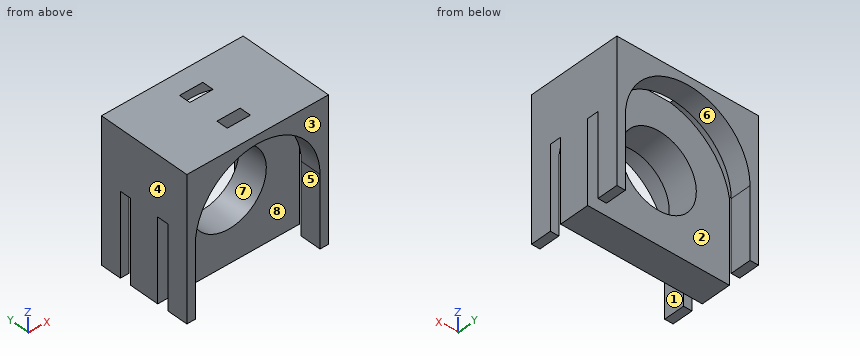
from build123d import *

# Parameters (mm, degrees)
SKETCH1_W           = 15
SKETCH1_H           = 15
BOSS_EXTRUDE1_DEPTH = 5
SKETCH2_W           = 15
SKETCH2_H           = 2.5
BOSS_EXTRUDE2_DEPTH = 15
CUT_EXTRUDE1_START  = -7.5
CUT_EXTRUDE1_DEPTH  = 31
SKETCH4_R           = 7.6
CUT_EXTRUDE2_DEPTH  = 1.2
SKETCH5_R           = 6.6
CUT_EXTRUDE3_DEPTH  = 23.2125
CUT_EXTRUDE4_START  = 1.2
SKETCH6_R           = 7.6
CUT_EXTRUDE4_DEPTH  = 1.2
SKETCH7_R           = 6.6
CUT_EXTRUDE5_DEPTH  = 23.2125
SKETCH8_R           = 4
CUT_EXTRUDE6_DEPTH  = 23.2125


with BuildPart() as part:
    # Sketch1 → Boss-Extrude1 (new body)
    with BuildSketch(Plane(origin=(0, 0, 0), x_dir=(1, 0, 0), z_dir=(0, 1, 0))):
        with Locations((7.5, -7.5)):
            Rectangle(SKETCH1_W, SKETCH1_H)
    extrude(amount=BOSS_EXTRUDE1_DEPTH)

    # Sketch2 → Boss-Extrude2 (add)
    with BuildSketch(Plane.XY.offset(15)):
        with Locations((7.5, 6.25)):
            Rectangle(SKETCH2_W, SKETCH2_H)
        with Locations((7.5, -1.25)):
            Rectangle(SKETCH2_W, SKETCH2_H)
    extrude(amount=-BOSS_EXTRUDE2_DEPTH)

    # Sketch3 → Cut-Extrude1 (cut)
    with BuildSketch(Plane(origin=(0, 0, 0), x_dir=(-1, 0, 0), z_dir=(0, 0, -1)).offset(CUT_EXTRUDE1_START)):
        Polygon((-14.1, 7.5), (-14.1, 5.2875), (-15.1, 5.2875), (-15.1, 4.0875), (-7.5, 4.0875), (0.1, 4.0875), (0.1, 5.2875), (-0.9, 5.2875), (-0.9, 7.5), align=None)
    cut_extrude1 = extrude(amount=CUT_EXTRUDE1_DEPTH, mode=Mode.SUBTRACT)

    # Sketch4 → Cut-Extrude2 (cut)
    with BuildSketch(Plane(origin=(0, 4.0875, 0), x_dir=(1, 0, 0), z_dir=(0, 1, 0))):
        with Locations((7.5, -7.5)):
            Circle(SKETCH4_R)
    extrude(amount=CUT_EXTRUDE2_DEPTH, mode=Mode.SUBTRACT)

    # Sketch5 → Cut-Extrude3 (cut, through all)
    with BuildSketch(Plane(origin=(0, 4.0875, 0), x_dir=(1, 0, 0), z_dir=(0, 1, 0))):
        with Locations((7.5, -7.5)):
            Circle(SKETCH5_R)
    extrude(amount=CUT_EXTRUDE3_DEPTH, mode=Mode.SUBTRACT)

    # Mirror1: Cut-Extrude1 across plane
    add(cut_extrude1.mirror(Plane(origin=(0, 2.5, 0), x_dir=(0, 0, 1), z_dir=(0, -1, 0))), mode=Mode.SUBTRACT)

    # Sketch6 → Cut-Extrude4 (cut)
    with BuildSketch(Plane.XZ.offset(-0.9125).offset(CUT_EXTRUDE4_START)):
        with Locations((7.5, 7.5)):
            Circle(SKETCH6_R)
    extrude(amount=-CUT_EXTRUDE4_DEPTH, mode=Mode.SUBTRACT)

    # Sketch7 → Cut-Extrude5 (cut, through all)
    with BuildSketch(Plane.XZ.offset(-0.9125)):
        with Locations((7.5, 7.5)):
            Circle(SKETCH7_R)
    extrude(amount=CUT_EXTRUDE5_DEPTH, mode=Mode.SUBTRACT)

    # Sketch8 → Cut-Extrude6 (cut, through all)
    with BuildSketch(Plane(origin=(0, 4.0875, 0), x_dir=(1, 0, 0), z_dir=(0, 1, 0))):
        with Locations(Location((7.5, -7.5, 0), (0, 0, 270))):
            Circle(SKETCH8_R)
    extrude(amount=-CUT_EXTRUDE6_DEPTH, mode=Mode.SUBTRACT)


solid = part.part
For this review, take the finished solid that the model builds, in its own axes (mm). Face numbers are marked on the shaded views. A direction names the side the tool comes from. Round coordinates to 2 decimals unless told otherwise and drop trailing zeros. Write each loop counter-clockwise with the first axis right and the second up, starting at its lowest first coordinate (ties: lowest second). Pieces come first, ordered by that corner, then holes. Notation, with made-up numbers: (52, -12.75) - (87, -12.75) arc R5 ccw to (87, -4.75) - close; hole circle Ø2 at (45.5, 31.25). An arc over 180 degrees is marked (long way). Write item = value, one per line. Start each with the question number.
1. Wall thickness on L1, parallel to X at y = 5.5, z = 4.75; L2, parallel to X at y = 2.5, z = 7.5; L3, parallel to Y at x = 13.5, z = 4.5: over which ranges is each line inside the solid? List them lowest first.
2. Consider section D-D on y = 0.25. State the section outline as (x, z) points.
3. Consider section A-A on x = 7.5. State the section outline as (y, z) points.
4. Draft analysis for pull direction Y (two halves, no side actions). For the marked faces 1, 2 and 3, state which applies: released by +Y, released by -Y, zero draft, split by the parting line, or undercut.
5. Consider section C-C on x = 5.5. State the section outline as (y, z) points, plus the area to 3 significant figures.
6. Consider section B-B on z = 10.25. State the section outline as (x, y) points.
7. For pin 1 Ø9 at (x, z) = (7.5, 7.5) entering from +Y; pin 2 Ø4.5 at (x, z) = (6, 9) entering from -Y, all flat-tipped, find the tip position at first contact; note any pin that passes through.
8. For the marked faces 4, 5, 6, 7 and 8, list the 3-axis set-ups (+Z, -Z, +X, -X, +Y, -Y) from which the entire face can be reached by the end or side of a thin tool; tool diameter is ignored.
Evaluation:
q1.L1 = 0 to 0.9, 14.1 to 15
q1.L2 = 0 to 3.5, 11.5 to 15
q1.L3 = 0.91 to 4.09
q2.outline = (0, 8.73) arc R7.6 cw to (6.27, 15) - (0, 15) - close; (8.73, 15) arc R7.6 cw to (15, 8.73) - (15, 15) - close
q3.outline = (-2.5, 14.1) - (-0.29, 14.1) - (-0.29, 15) - (-2.5, 15) - close; (0.91, 0) - (4.09, 0) - (4.09, 3.5) - (0.91, 3.5) - close; (0.91, 11.5) - (4.09, 11.5) - (4.09, 15) - (0.91, 15) - close; (5.29, 14.1) - (7.5, 14.1) - (7.5, 15) - (5.29, 15) - close
q4.face_1 = zero draft
q4.face_2 = undercut
q4.face_3 = released by -Y
q5.outline = (-2.5, 13.79) - (-0.29, 13.79) - (-0.29, 14.83) - (0.91, 14.83) - (0.91, 10.96) - (4.09, 10.96) - (4.09, 14.83) - (5.29, 14.83) - (5.29, 13.79) - (7.5, 13.79) - (7.5, 15) - (-2.5, 15) - close; (0.91, 0) - (4.09, 0) - (4.09, 4.04) - (0.91, 4.04) - close
q5.area = 31.4 mm2
q6.outline = (0, -2.5) - (1.5, -2.5) - (1.5, -0.29) - (0.41, -0.29) - (0.41, 0.91) - (4.6, 0.91) - (4.6, 4.09) - (0.41, 4.09) - (0.41, 5.29) - (1.5, 5.29) - (1.5, 7.5) - (0, 7.5) - close; (10.4, 0.91) - (14.59, 0.91) - (14.59, -0.29) - (13.5, -0.29) - (13.5, -2.5) - (15, -2.5) - (15, 7.5) - (13.5, 7.5) - (13.5, 5.29) - (14.59, 5.29) - (14.59, 4.09) - (10.4, 4.09) - close
q7.pin_1 = 4.09
q7.pin_2 = 0.91
q8.face_4 = +Z, -Z, -X, +Y, -Y
q8.face_5 = -Z, -Y
q8.face_6 = -Z, +Y
q8.face_7 = +Y, -Y
q8.face_8 = -Z
